from build123d import *

# Parameters (mm, degrees)
BOSS_EXTRUDE1_DEPTH = 10
SKETCH2_W           = 14
SKETCH2_H           = 10
SKETCH2_R           = 2.25
BOSS_EXTRUDE2_DEPTH = 4
FILLET1_R           = 2


with BuildPart() as part:
    # Sketch1 → Boss-Extrude1 (new body, symmetric)
    with BuildSketch(Plane.XY):
        with BuildLine():
            Line((-13.919410907, 1.5), (-9.886859967, 1.5))
            ThreePointArc((-9.886859967, 1.5), (0, 10), (9.886859967, 1.5))
            Line((9.886859967, 1.5), (13.919410907, 1.5))
            ThreePointArc((13.919410907, 1.5), (0, 14), (-13.919410907, 1.5))
        make_face()
    extrude(amount=BOSS_EXTRUDE1_DEPTH, both=True)

    # Sketch2 → Boss-Extrude2 (add)
    with BuildSketch(Plane.XZ.offset(-1.5)):
        with Locations((16.886859967, 0)):
            Rectangle(SKETCH2_W, SKETCH2_H)
        with Locations((18.903135437, 0)):
            Circle(SKETCH2_R, mode=Mode.SUBTRACT)
        with Locations((-16.886859967, 0)):
            Rectangle(SKETCH2_W, SKETCH2_H)
        with Locations((-18.903135437, 0)):
            Circle(SKETCH2_R, mode=Mode.SUBTRACT)
    extrude(amount=-BOSS_EXTRUDE2_DEPTH)

    # Fillet1
    fillet1_edges = [part.edges().sort_by_distance(p)[0] for p in [
        (-12.87439319, 5.5, 0),
        (12.87439319, 5.5, 0),
        (13.54536764, 3.538787293, -5),
        (13.54536764, 3.538787293, 5),
        (23.886859967, 3.5, 5),
        (23.886859967, 3.5, -5),
        (-23.886859967, 3.5, 5),
        (-13.54536764, 3.538787293, -5),
        (-23.886859967, 3.5, -5),
        (-13.54536764, 3.538787293, 5),
    ]]
    fillet(fillet1_edges, radius=FILLET1_R)


solid = part.part
Can you work these out from the model? Positions are in its coordinate system, mm. A direction names the side the tool comes from. Coordinates: 2 decimals unless noted, no trailing zeros. Write each loop counter-clockwise with the first axis right and the second up, starting at its lowest first coordinate (ties: lowest second). Pieces come first, ordered by that corner, then holes. Notation, with made-up numbers: (9.25, 14) -> (50.25, 14) arc R22 ccw to (50.25, 43) -> close; hole circle Ø8 at (83, -28.75). An arc over 180 degrees is marked (long way). Write each question's results on one line, items separated by ' | '. Start each with the question number.
Q1. Imagine slicing it at B-B (y = 7). Write out the boundary of the cut face in (x, z).
Q2. We'd pull the mould along Z, two halves only. Please class faces 1 (the face through (-23.887, 3, 0)), 2 (the face through (-23.317, 3.528, 4.399)), 3 (the face through (-20.56, 3.47, 1.52)): +Z half, -Z half, draft (parallel to the pull), parting line (faces both ways), or undercut.
Q3. On a 3-axis mill with a long thin cutter (end or side, diameter ignored), from which of +Z, -Z, +X, -X, +Y, -Y can I reach the whole of each face in a straight line? I mean faces 4 (the face through (18.9, 5.5, 2.4)), 5 (the face through (-15, 1.5, 0)), 6 (the face through (-19.1, 5.5, 2.4)). Say none if no direction works.
Q4. Imagine slicing it at C-C (z = 4). Write out the boundary of the cut face in (x, y).
Q5. If I drill on probe 1 along X at (y, z) = (3.5, -0.25); probe 2 along Y at (x, z) = (-22, 1.5); probe 3 along X at (y, z) = (3, 0.75), over which ranges is the centre line in solid material (lowest first)?
Q6. Imagine slicing it at D-D (y = 4.5). State how many separate pieces and enclosed holes the cut face has, then the cut area to 3 significant figures.
Q7. I'm going to push flat-ended pins straight in: pin 1 (2 mm diameter, centred on y = 8.5, z = 0, fed in from -X); pin 2 (10.5 mm diameter, centred on x = 20.5, z = -1, fed in from +Y); pin 3 (2 mm diameter, centred on x = 19, y = 4.5, fed in from +Z). Where does each tip first touch, or does it pass through?
Q8. Imagine slicing it at A-A (z = 0). Write out the boundary of the cut face in (x, y), then the cut area to 3 significant figures.
Taken from the geometry:
1) outline: (-12.12, -10) -> (-7.14, -10) -> (-7.14, 10) -> (-12.12, 10) -> close; (7.14, -10) -> (12.12, -10) -> (12.12, 10) -> (7.14, 10) -> close
2) face 1: draft | face 2: +Z half | face 3: undercut
3) face 4: +Z, -Z, +X, +Y | face 5: +Z, -Z, +X, -X, -Y | face 6: +Z, -Z, -X, +Y
4) outline: (-23.62, 1.5) -> (-9.89, 1.5) arc R10 cw to (9.89, 1.5) -> (23.62, 1.5) -> (23.62, 5.5) -> (14.13, 5.5) arc R2 cw to (12.37, 6.56) arc R14 ccw to (-12.37, 6.56) arc R2 cw to (-14.13, 5.5) -> (-23.62, 5.5) -> close
5) probe 1: x = -23.89 to -21.14, -16.67 to -9.37, 9.37 to 16.67, 21.14 to 23.89 | probe 2: y = 1.5 to 5.5 | probe 3: x = -23.89 to -21.02, -16.78 to -9.54, 9.54 to 16.78, 21.02 to 23.89
6) separate pieces: 2 | enclosed holes: 2 | area: 354 mm^2
7) pin 1: stops at x = -11.82 | pin 2: stops at y = 5.5 | pin 3: stops at z = 5
8) outline: (-23.89, 1.5) -> (-21.15, 1.5) -> (-21.15, 5.5) -> (-23.89, 5.5) -> close; (-16.65, 1.5) -> (-9.89, 1.5) arc R10 cw to (9.89, 1.5) -> (16.65, 1.5) -> (16.65, 5.5) -> (14.13, 5.5) arc R2 cw to (12.37, 6.56) arc R14 ccw to (-12.37, 6.56) arc R2 cw to (-14.13, 5.5) -> (-16.65, 5.5) -> close; (21.15, 1.5) -> (23.89, 1.5) -> (23.89, 5.5) -> (21.15, 5.5) -> close | area: 186 mm^2
